The drawing under review shows one solid part. Ordinate dimensions are in mm from its lowest x, y, z. Give positions to 0.01 mm unless a question says otherwise; leave off trailing zeros. Loops run counter-clockwise (first coordinate to the right, second up) from the corner with the lowest first, then second, coordinate; pieces in that order, holes last. Notation, with made-up numbers: (-14, 40) -> (-1, 40) arc R31 cw to (-1, 79) -> close; hole circle Ø4 at (62.25, -18). An arc over 180 degrees is marked (long way). Answer in a Markdown table with one row per item. Add a question column.
(1) Consider section A-A on x = 72. Write out the cut boundary in (y, z), then the cut area to 3 significant figures.
(2) Consider section B-B on y = 72. Write out the cut boundary in (x, z).
(3) For line 1 (Y direction, x = 72, z = 0.7); line 2 (Y direction, x = 18.5, z = 0.9) (1 decimal); line 3 (X direction, y = 134, z = 0.7) (1 decimal), list the stretches that pass through material, from the lowest coordinate up.
(4) Consider section D-D on y = 8. Write out the cut boundary in (x, z) (1 decimal).
(5) For pin 1 (0.9 mm diameter, centred on x = 67.5, z = 1.5, fed in from +Y), flat-tipped, find the tip position at first contact; note if it passes through.
(6) Consider section C-C on z = 0.55. Write out the cut boundary in (x, y).
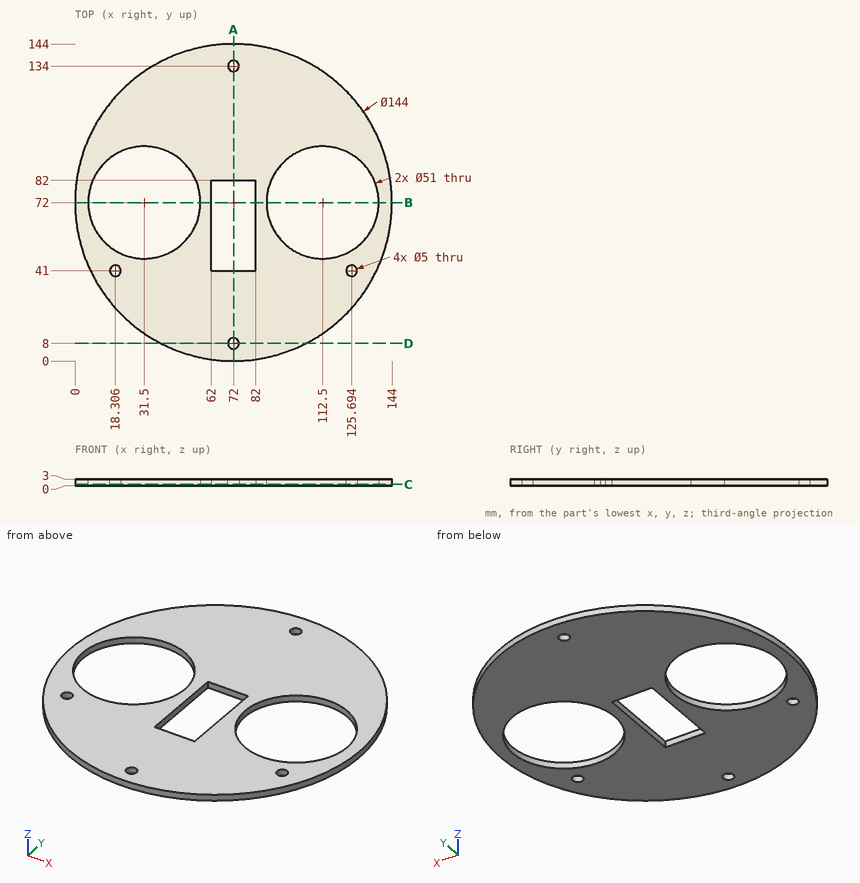
Values follow:
| question | item | result |
|---|---|---|
| 1 | outline | (0, 0) -> (5.5, 0) -> (5.5, 3) -> (0, 3) -> close; (10.5, 0) -> (41, 0) -> (41, 3) -> (10.5, 3) -> close; (82, 0) -> (131.5, 0) -> (131.5, 3) -> (82, 3) -> close; (136.5, 0) -> (144, 0) -> (144, 3) -> (136.5, 3) -> close |
| 1 | area | 279 mm2 |
| 2 | outline | (0, 0) -> (6, 0) -> (6, 3) -> (0, 3) -> close; (57, 0) -> (62, 0) -> (62, 3) -> (57, 3) -> close; (82, 0) -> (87, 0) -> (87, 3) -> (82, 3) -> close; (138, 0) -> (144, 0) -> (144, 3) -> (138, 3) -> close |
| 3 | line 1 | 0 to 5.5, 10.5 to 41, 82 to 131.5, 136.5 to 144 |
| 3 | line 2 | 23.8 to 38.5, 43.5 to 50.1, 93.9 to 120.2 |
| 3 | line 3 | 35.4 to 69.5, 74.5 to 108.6 |
| 4 | outline | (39, 0) -> (69.5, 0) -> (69.5, 3) -> (39, 3) -> close; (74.5, 0) -> (105, 0) -> (105, 3) -> (74.5, 3) -> close |
| 5 | pin 1 | y = 143.89 |
| 6 | outline | circle Ø144 at (72, 72); hole circle Ø51 at (31.5, 72); hole circle Ø5 at (18.31, 41); hole (62, 41) -> (82, 41) -> (82, 82) -> (62, 82) -> close; hole circle Ø5 at (72, 8); hole circle Ø5 at (72, 134); hole circle Ø51 at (112.5, 72); hole circle Ø5 at (125.69, 41) |
